Drawing for the job (mm, zero at the part's lowest x, y, z). A direction names the side the tool comes from. Give positions to 0.01 mm unless a question says otherwise; leave off trailing zeros. Order: outer loops, then holes, each group sorted by start corner. A loop starts at its lowest first (then second) coordinate and runs counter-clockwise, first axis right, second up. Notation, with made-up numbers: M 23.25,8 L 29.25,8 A28 cw 29.25,32 Z; hole C -36,25 d10. An arc over 180 degrees is marked long. Answer as a JSON object with one key per item and string values.
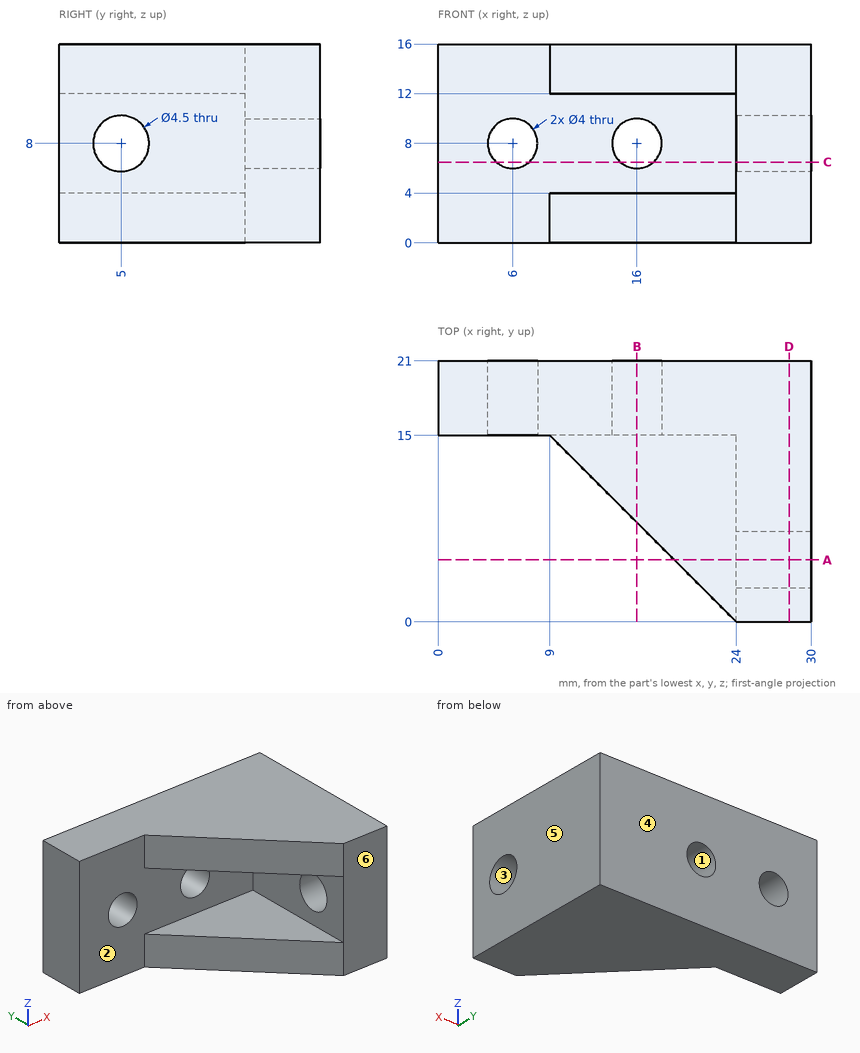
1. Cut at D-D on x = 28.25. Give the cut face in (y, z), plus the area to 3 significant figures.
Worked answers:
{"outline": "M 0,0 L 21,0 L 21,16 L 0,16 Z; hole C 5,8 d4.5", "area": "320 mm^2"}
2. Pin check, flat tips, straight feed: P1, Ø2.5, axis at x = 6, z = 8, coming from the -Y side; P2, Ø5, axis at x = 3, z = 4, coming from the -Y side. Stop position of each tip, or through.
Worked answers:
{"P1": "passes through", "P2": "stops at y = 15"}
3. Two-plate mould, pull along Y, no slides. Class the marked faces 3, 4, 5 and 6: +Y half, -Y half, draft (parallel to the pull), parting line (faces both ways), or undercut.
Worked answers:
{"face 3": "undercut", "face 4": "+Y half", "face 5": "draft", "face 6": "-Y half"}
4. Probe line 1 along Z through (x, y) = (6, 18.6); line 2 along X through (y, z) = (16.5, 6.25); line 3 along Z through (x, y) = (26.5, 5). List the from-to ranges inside material, lowest first.
Worked answers:
{"line 1": "z = 0 to 6, 10 to 16", "line 2": "x = 0 to 5.03, 6.97 to 15.03, 16.97 to 30", "line 3": "z = 0 to 5.75, 10.25 to 16"}
5. Cut at A-A on y = 5. Give the cut face in (x, z), plus the area to 3 significant figures.
Worked answers:
{"outline": "M 19,0 L 30,0 L 30,5.75 L 24,5.75 L 24,4 L 19,4 Z; M 19,12 L 24,12 L 24,10.25 L 30,10.25 L 30,16 L 19,16 Z", "area": "109 mm^2"}
6. Which spindle directions (+Z, -Z, +X, -X, +Y, -Y) get a long thin tool onto all of the face, cutting with end or side? Do the marked faces 1 and 2. Say none if no direction does.
Worked answers:
{"face 1": "+Y, -Y", "face 2": "-X, -Y"}
7. Cut at C-C on z = 6.5. Give the cut face in (x, y), plus the area to 3 significant figures.
Worked answers:
{"outline": "M 0,15 L 4.68,15 L 4.68,21 L 0,21 Z; M 7.32,15 L 14.68,15 L 14.68,21 L 7.32,21 Z; M 17.32,15 L 24,15 L 24,6.68 L 30,6.68 L 30,21 L 17.32,21 Z; M 24,0 L 30,0 L 30,3.32 L 24,3.32 Z", "area": "218 mm^2"}
8. Cut at B-B on x = 16. Give the cut face in (y, z).
Worked answers:
{"outline": "M 8,0 L 21,0 L 21,6 L 15,6 L 15,4 L 8,4 Z; M 8,12 L 15,12 L 15,10 L 21,10 L 21,16 L 8,16 Z"}
